For this review, take the finished solid that the model builds, in its own axes (mm). Give positions to 0.01 mm unless a question says otherwise; leave off trailing zeros. Loops run counter-clockwise (first coordinate to the right, second up) from the corner with the lowest first, then second, coordinate; pieces in that order, holes last.
```python
from build123d import *

# Parameters (mm, degrees)
SKETCH1_R           = 3.96875
BOSS_EXTRUDE1_DEPTH = 333.375
SKETCH2_R           = 2.032
CUT_EXTRUDE1_DEPTH  = 12.7
CUT_EXTRUDE2_START  = -12.7
SKETCH3_R           = 2.032
CUT_EXTRUDE2_DEPTH  = 12.7
CHAMFER1_SIZE       = 0.254


with BuildPart() as part:
    # Sketch1 → Boss-Extrude1 (new body)
    with BuildSketch(Plane.XY):
        Circle(SKETCH1_R)
    extrude(amount=BOSS_EXTRUDE1_DEPTH)

    # Sketch2 → Cut-Extrude1 (cut)
    with BuildSketch(Plane.XY.offset(333.375)):
        Circle(SKETCH2_R)
    extrude(amount=-CUT_EXTRUDE1_DEPTH, mode=Mode.SUBTRACT)

    # Sketch3 → Cut-Extrude2 (cut)
    with BuildSketch(Plane(origin=(0, 0, 0), x_dir=(-1, 0, 0), z_dir=(0, 0, -1)).offset(CUT_EXTRUDE2_START)):
        with Locations(Location((0, 0, 0), (0, 0, 180))):
            Circle(SKETCH3_R)
    extrude(amount=CUT_EXTRUDE2_DEPTH, mode=Mode.SUBTRACT)

    # Chamfer1
    chamfer1_edges = [part.edges().sort_by_distance(p)[0] for p in [
        (-2.032, 0, 0),
        (-3.96875, 0, 0),
        (-3.96875, 0, 333.375),
        (-2.032, 0, 333.375),
    ]]
    chamfer(chamfer1_edges, length=CHAMFER1_SIZE)


solid = part.part
```
Q1. Consider section C-C on z = 151.5. Give the boundary of the cut face in (x, y).
Answers:
outline: circle Ø7.94 at (0, 0)
Q2. For pin 1 Ø2 at (x, z) = (2, 265.5) entering from +Y; pin 2 Ø1.2 at (x, y) = (0, 0.5) entering from +Z (3 decimals); pin 3 Ø2 at (x, y) = (-0.5, 0) entering from -Z, all flat-tipped, find the tip position at first contact; note any pin that passes through.
Answers:
pin 1: stops at y = 3.84
pin 2: stops at z = 320.675
pin 3: stops at z = 12.7
Q3. Consider section A-A on x = 0. Give the boundary of the cut face in (y, z) (3 decimals).
Answers:
outline: (-3.969, 0.254) - (-3.715, 0) - (-2.286, 0) - (-2.032, 0.254) - (-2.032, 12.7) - (2.032, 12.7) - (2.032, 0.254) - (2.286, 0) - (3.715, 0) - (3.969, 0.254) - (3.969, 333.121) - (3.715, 333.375) - (2.286, 333.375) - (2.032, 333.121) - (2.032, 320.675) - (-2.032, 320.675) - (-2.032, 333.121) - (-2.286, 333.375) - (-3.715, 333.375) - (-3.969, 333.121) - close
Q4. For probe 1 along Y at (x, z) = (0, 324.5); probe 2 along Z at (x, y) = (2, 1); probe 3 along Y at (x, z) = (0.25, 318), list the stretches that pass through material, from the lowest coordinate up.
Answers:
probe 1: y = -3.97 to -2.03, 2.03 to 3.97
probe 2: z = 0.05 to 333.33
probe 3: y = -3.96 to 3.96
